For this review, use the dimensioned drawing (mm, ordinates from the lowest corner) and the shaded views. Round coordinates to 2 decimals unless told otherwise and drop trailing zeros. Order: outer loops, then holes, each group sorted by start corner. A loop starts at its lowest first (then second) coordinate and runs counter-clockwise, first axis right, second up. Notation, with made-up numbers: (33.25, 86.5) -> (44.25, 86.5) arc R25 cw to (44.25, 109.5) -> close; hole circle Ø11 at (-38.5, -11). An arc over 180 degrees is marked (long way). Answer in a Markdown table with one row per item.
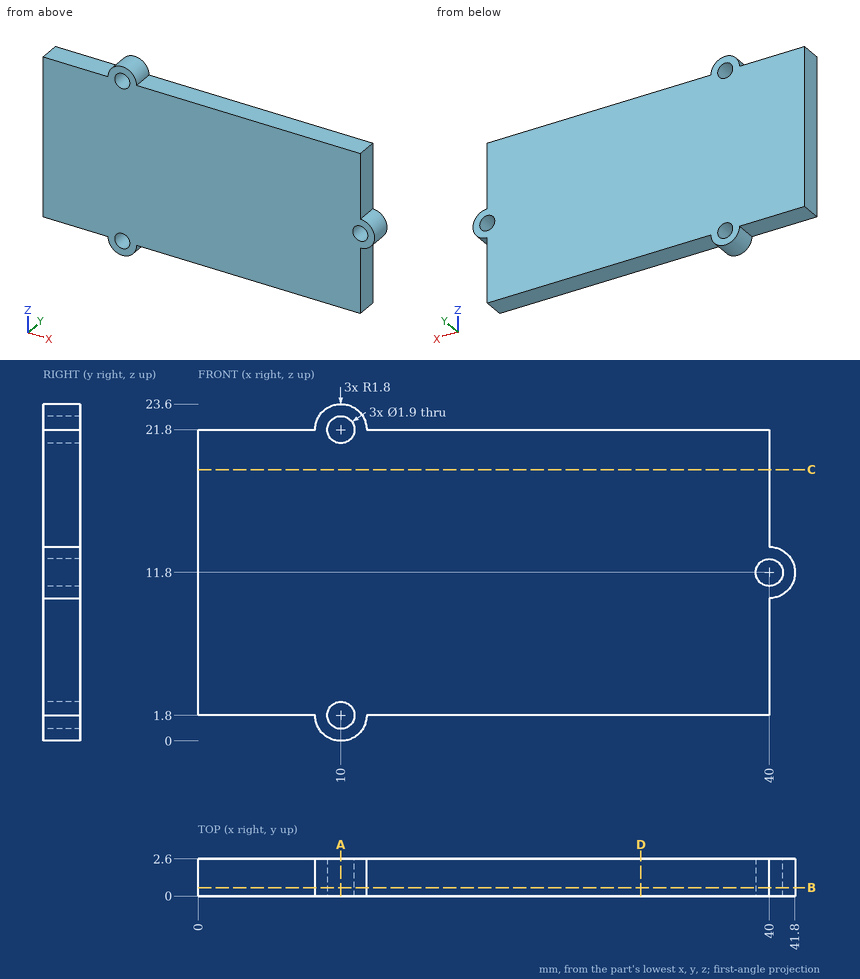
Q1. Take a section at B-B, the plane y = 0.6. Write out the cut boundary in (x, z).
Answer key:
| item | result |
|---|---|
| outline | (0, 1.8) -> (8.2, 1.8) arc R1.8 ccw to (11.8, 1.8) -> (40, 1.8) -> (40, 10) arc R1.8 ccw to (40, 13.6) -> (40, 21.8) -> (11.8, 21.8) arc R1.8 ccw to (8.2, 21.8) -> (0, 21.8) -> close; hole circle Ø1.9 at (10, 1.8); hole circle Ø1.9 at (10, 21.8); hole circle Ø1.9 at (40, 11.8) |
Q2. To check wall thickness, follow probe 1 along Z at (x, y) = (10, 1.5); probe 2 along X at (y, z) = (1.15, 11.8); probe 3 along Z at (x, y) = (3, 0.8). State the ranges of each line that lie inside material, in increasing order.
Answer key:
| item | result |
|---|---|
| probe 1 | z = 0 to 0.85, 2.75 to 20.85, 22.75 to 23.6 |
| probe 2 | x = 0 to 39.05, 40.95 to 41.8 |
| probe 3 | z = 1.8 to 21.8 |
Q3. Take a section at C-C, the plane z = 19. Write out the cut boundary in (x, y), then the cut area to 3 significant figures.
Answer key:
| item | result |
|---|---|
| outline | (0, 0) -> (40, 0) -> (40, 2.6) -> (0, 2.6) -> close |
| area | 104 mm^2 |
Q4. Clearance check with flat-ended pins moving along their axes: pin 1 Ø0.8 at (y, z) = (1.5, 4.5) entering from +X; pin 2 Ø0.8 at (x, y) = (25.5, 2) entering from +Z; pin 3 Ø1.5 at (x, z) = (40, 11.8) entering from +Y; pin 4 Ø1.5 at (x, y) = (24, 1) entering from -Z. State where each tip first meets the part, or that it passes through.
Answer key:
| item | result |
|---|---|
| pin 1 | stops at x = 40 |
| pin 2 | stops at z = 21.8 |
| pin 3 | passes through |
| pin 4 | stops at z = 1.8 |
Q5. Take a section at D-D, the plane x = 31. Write out the cut boundary in (y, z).
Answer key:
| item | result |
|---|---|
| outline | (0, 1.8) -> (2.6, 1.8) -> (2.6, 21.8) -> (0, 21.8) -> close |
Q6. Take a section at A-A, the plane x = 10. Write out the cut boundary in (y, z).
Answer key:
| item | result |
|---|---|
| outline | (0, 0) -> (2.6, 0) -> (2.6, 0.85) -> (0, 0.85) -> close; (0, 2.75) -> (2.6, 2.75) -> (2.6, 20.85) -> (0, 20.85) -> close; (0, 22.75) -> (2.6, 22.75) -> (2.6, 23.6) -> (0, 23.6) -> close |
